Verification items for the finished model (mm, model axes). Face numbers are marked on the shaded views. A direction names the side the tool comes from. Round coordinates to 2 decimals unless told otherwise and drop trailing zeros. Order: outer loops, then holes, each group sorted by start corner. A loop starts at its lowest first (then second) coordinate and runs counter-clockwise, first axis right, second up. Notation, with made-up numbers: (47.5, 3.5) -> (67.5, 3.5) arc R18 cw to (67.5, 13.5) -> close; hole circle Ø6 at (43, 9). An arc over 180 degrees is marked (long way). Return JSON: item names as keys, results as strings. Group by question number.
Item 1: Sectioned sample at D-D on z = -12.5. Record the cut outline in (x, y) (3 decimals), plus the area to 3 significant figures.
Item 2: Depth check by flat-ended pin: pin 1 Ø1.7 at (y, z) = (12, 3) entering from +X; pin 2 Ø12 at (y, z) = (-6.5, -9.5) entering from -X (3 decimals); pin 3 Ø6 at (x, z) = (0, -13.14) entering from +Y (3 decimals); pin 4 Ø3 at (x, z) = (-10, -3) entering from -Y. Enter the tip coordinate at first touch or a pass-through.
Item 3: Sectioned sample at B-B on y = 1.5. Give the number of separate pieces and of enclosed holes in the cut face, plus the area to 3 significant figures.
Item 4: Scan lines: probe 1 along Z at (x, y) = (0, 0.5); probe 2 along X at (y, z) = (-2, -12) (3 decimals); probe 3 along Z at (x, y) = (-3, -11.5). Record each from-to range of solid material in increasing order. Write a range as from..to.
Item 5: Draft check along Z on the marked faces 1, 2, 3 and 4. Enter one of: pulls with the +Z half, pulls with the -Z half, needs draft (parallel to the pull), parting line crosses it, or undercut.
Item 6: Access from +Z, -Z, +X, -X, +Y, -Y to the whole of each face (thin tool, end or side, straight path). Record for the marked faces 5, 6 and 7.
Item 7: Sectioned sample at A-A on z = -2.75. Record the cut outline in (x, y) (3 decimals).
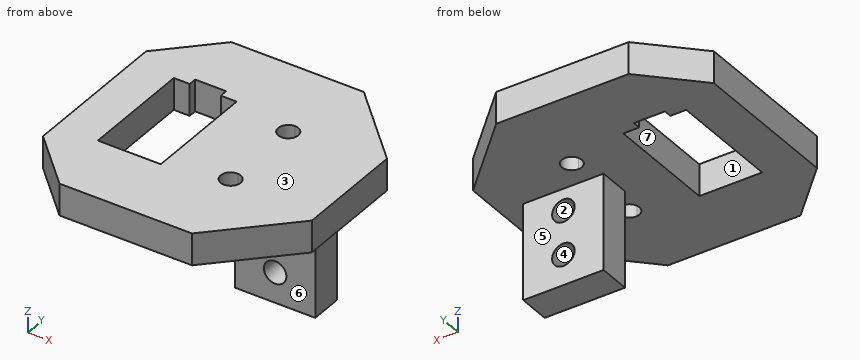
Autodesk Inventor part; units mm, degrees
ref_plane "YZ Plane" through (0, 0, 0) normal (1, 0, 0) x (0, 1, 0)
ref_plane "XZ Plane" through (0, 0, 0) normal (0, 1, 0) x (-1, 0, 0)
ref_plane "XY Plane" through (0, 0, 0) normal (0, 0, 1) x (1, 0, 0)
sketch "Sketch1" plane through (0, 0, 0) normal (0, 0, 1) x (1, 0, 0)
  line L0 (-38.1, -25.4) -> (38.1, -25.4)
  line L1 (38.1, -25.4) -> (38.1, 25.4)
  line L2 (38.1, 25.4) -> (-38.1, 25.4)
  line L3 (-38.1, 25.4) -> (-38.1, -25.4)
  line L4 (-38.1, -25.4) -> (38.1, 25.4) construction
  line L5 (38.1, -25.4) -> (-38.1, 25.4) construction
  point P0 (0, 0)
  dimension "d0" = 76.2
  dimension "d1" = 50.8
extrude "Extrusion1" add sketch "Sketch1" along normal blind 6.35
sketch "Sketch3" plane through (38.1, -25.4, 0) normal (1, 0, 0) x (0, 0, -1)
  line L0 (0, 0) -> (0, 50.8)
  line L1 (0, 50.8) -> (-6.35, 50.8)
  line L2 (-6.35, 0) -> (-6.35, 50.8)
  line L3 (0, 0) -> (-6.35, 0)
  point P0 (0, 25.4)
extrude "Extrusion3" cut sketch "Sketch3" against normal blind 25.4
sketch "Sketch4" plane through (-38.1, -25.4, 0) normal (-1, 0, 0) x (0, 0, 1)
  line L0 (4.925, 17.15) -> (1.425, 17.15)
  line L1 (1.425, 17.15) -> (1.425, 33.65)
  line L2 (1.425, 33.65) -> (4.925, 33.65)
  line L3 (4.925, 33.65) -> (4.925, 17.15)
  line L4 (4.925, 17.15) -> (1.425, 33.65) construction
  line L5 (1.425, 17.15) -> (4.925, 33.65) construction
  point P0 (0, 25.4)
  point P1 (3.175, 25.4)
  dimension "d9" = 3.5
  dimension "d10" = 16.5
extrude "Extrusion4" add sketch "Sketch4" along normal blind 3.302
sketch "Sketch5" plane through (-38.1, -8.25, 4.925) normal (0, 0, 1) x (1, 0, 0)
  line L0 (-3.302, 0) -> (-3.302, 16.5)
  line L1 (0, 16.5) -> (0, 0)
  line L2 (0, 16.5) -> (-3.302, 16.5)
  line L3 (-3.302, 0) -> (-3.302, 16.5)
  line L4 (0, 0) -> (-3.302, 0)
  line L5 (-3.302, 16.5) -> (-3.175, 16.5)
  line L6 (0, 16.5) -> (-3.302, 16.5)
  line L7 (-3.175, 16.5) -> (-3.175, 16.5685)
  line L8 (-3.302, 16.5) -> (-3.302, 0)
  line L9 (-3.175, 16.5685) -> (-3.302, 16.5)
  point P0 (38.1, 8.25)
  point P1 (-3.175, 16.5)
  dimension "d13" = 0.127
sketch3d "3D Sketch1"
  line L0 (-41.402, 8.25, 4.925) -> (-41.402, 8.25, 1.425)
  line L1 (-41.402, 8.25, 1.425) -> (-41.402, -8.25, 1.425)
  line L2 (-41.402, -8.25, 1.425) -> (-41.402, -8.25, 4.925)
  line L3 (-41.402, -8.25, 4.925) -> (-41.402, 8.25, 4.925)
sweep "Sweep1" add profiles "Sketch5" path "3D Sketch1" contours L9 L7 L2
chamfer "Chamfer1" distance 14.2875 angle 45 4 edges at (-38.1, -25.4, 3.175) (-38.1, 25.4, 3.175) (12.7, -25.4, 3.175) (12.7, 25.4, 3.175)
sketch "Sketch6" plane through (-41.402, -25.4, 0) normal (-1, 0, 0) x (0, 0, 1)
  line L0 (-26.5368, -66.9991) -> (26.5368, -66.9991)
  line L1 (26.5368, -66.9991) -> (26.5368, 66.9991)
  line L2 (26.5368, 66.9991) -> (-26.5368, 66.9991)
  line L3 (-26.5368, 66.9991) -> (-26.5368, -66.9991)
  line L4 (0, 0) -> (6.35, 0)
  line L5 (-26.5368, -66.9991) -> (26.5368, 66.9991) construction
  line L6 (26.5368, -66.9991) -> (-26.5368, 66.9991) construction
  point P0 (0, 25.4)
extrude "Extrusion5" cut sketch "Sketch6" against normal blind 28.575
sketch "Sketch7" plane through (0, 0, 0) normal (0, 0, -1) x (-1, 0, 0)
  line L0 (-8.025, 3.175) -> (-8.025, -3.175)
  line L1 (-8.025, -3.175) -> (8.025, -3.175)
  line L2 (8.025, -3.175) -> (8.025, 3.175)
  line L3 (8.025, 3.175) -> (-8.025, 3.175)
  line L4 (-8.025, 4.675) -> (8.025, -1.675) construction
  line L5 (-8.025, -1.675) -> (8.025, 4.675) construction
  line L6 (0, 3.175) -> (0, -3.175)
  point P0 (0, 0)
  point P1 (0, 0)
  dimension "d21" = 6.35
  dimension "d22" = 16.05
extrude "Extrusion6" add sketch "Sketch7" along normal blind 19.2024
sketch "Sketch9" plane through (0, 0, 6.35) normal (0, 0, 1) x (1, 0, 0)
  line L0 (6.0307, -10.9832) -> (5.9693, 11.0167)
  line L1 (-6.0307, 10.9832) -> (6.0307, 10.9832)
  line L2 (6.0307, 10.9832) -> (6.0307, -10.9832)
  line L3 (6.0307, -10.9832) -> (-6.0307, -10.9832)
  line L4 (-6.0307, -10.9832) -> (-6.0307, 10.9832)
  point P0 (0, 0)
sketch "Sketch10" plane through (-12.827, -25.4, 0) normal (-1, 0, 0) x (0, 0, 1)
  line L0 (0, 0) -> (0, 50.8)
  line L1 (6.35, 0) -> (0, 0)
  line L2 (6.35, 50.8) -> (6.35, 0)
  line L3 (0, 50.8) -> (6.35, 50.8)
  point P0 (0, 25.4)
extrude "Extrusion7" add sketch "Sketch10" along normal blind 25.4
chamfer "Chamfer2" distance 10.16 angle 45 1 edges at (-38.227, 25.4, 3.175)
chamfer "Chamfer3" distance 10.16 angle 45 1 edges at (-38.227, -25.4, 3.175)
sketch "Sketch11" plane through (0, 0, 6.35) normal (0, 0, 1) x (1, 0, 0)
  line L0 (-29.728, 10.9832) -> (-17.6666, 10.9832)
  line L1 (-17.6666, -10.9832) -> (-29.728, -10.9832)
  line L2 (-29.728, -10.9832) -> (-29.728, 10.9832)
  line L3 (-17.6666, -10.9832) -> (-17.6666, 10.9832)
  line L4 (-30.998, 12.2532) -> (-16.3966, 12.2532)
  line L5 (-16.3966, 12.2532) -> (-16.3966, -12.2532)
  line L6 (-16.3966, -12.2532) -> (-30.998, -12.2532)
  line L7 (-30.998, -12.2532) -> (-30.998, 12.2532)
  line L8 (-17.6666, 10.9832) -> (-18.9366, 10.9832)
  line L9 (-29.728, 10.9832) -> (-28.458, 10.9832)
  line L10 (-18.9366, 10.9832) -> (-28.458, 10.9832)
  line L11 (-28.458, 10.9832) -> (-28.458, 15.1856)
  line L12 (-28.458, 15.1856) -> (-18.9366, 15.1856)
  line L13 (-18.9366, 15.1856) -> (-18.9366, 10.9832)
  point P0 (0, 0)
  dimension "d54" = 1.27
  dimension "d55" = 1.27
  dimension "d56" = 1.27
extrude "Extrusion8" cut sketch "Sketch11" against normal up to surface (6.35 mm away) contours L0 L3 L1 L2
sketch "Sketch12" plane through (0, 0, 6.35) normal (0, 0, 1) x (1, 0, 0)
  arc A0 (-5.2182, -6.4143) -> (-5.5402, -10.4006) centre (-5.418, -8.4043) ccw
  arc A1 (-5.5402, -10.4006) -> (-5.2182, -6.4143) centre (-5.3404, -8.4106) ccw
  arc A2 (-5.3792, 10.6071) -> (-5.3792, 6.6078) centre (-5.418, 8.6074) ccw
  arc A3 (-5.3792, 6.6078) -> (-5.3792, 10.6071) centre (-5.3404, 8.6074) ccw
  line L0 (-14.078, 16.1258) -> (3.242, 16.1258)
  line L1 (-14.078, 16.1258) -> (-14.078, -15.929)
  line L2 (-14.078, -15.929) -> (3.242, -15.929)
  line L3 (3.242, 16.1258) -> (3.242, -15.929)
  circle A4 centre (-5.3404, -8.4106) radius 2
  circle A5 centre (-5.3404, 8.6074) radius 2
  point P0 (0, 0)
  point P1 (-5.3792, 6.6078)
  point P2 (-5.2182, -6.4143)
  point P3 (-5.5402, -10.4006)
  dimension "d38" = 4
  dimension "d39" = 4
extrude "Extrusion9" cut sketch "Sketch12" against normal up to surface (6.35 mm away) contours A1 A4 | A3 A5
sketch "Sketch13" plane through (-8.025, 3.175, 0) normal (0, 1, 0) x (1, 0, 0)
  line L0 (16.05, 19.2024) -> (0, 19.2024)
  circle A0 centre (8.025, 4.3815) radius 2.25
  circle A1 centre (8.025, 13.1445) radius 2.25
  line L1 (16.05, 0) -> (0, 0)
  line L2 (16.05, 0) -> (16.05, 19.2024)
  line L3 (0, 19.2024) -> (16.05, 19.2024)
  line L4 (0, 0) -> (0, 19.2024)
  line L5 (8.025, 0) -> (12.4065, 0)
  line L6 (6.4375, 0) -> (20.725, 0)
  line L7 (8.025, 0) -> (8.025, 4.3815)
  line L8 (8.025, 0) -> (12.4065, 0) construction
  line L9 (8.025, 0) -> (21.1695, 0)
  line L10 (8.025, 0) -> (8.025, 13.1445)
  line L11 (16.05, 0) -> (0, 0)
  line L12 (8.025, 0) -> (21.1695, 0) construction
  dimension "d44" = 4.5
  dimension "d45" = 4.5
  dimension "d48" = 4.3815
  dimension "d49" = 4.3815
  dimension "d50" = 90
  dimension "d51" = 13.1445
  dimension "d52" = 13.1445
  dimension "d53" = 90
extrude "Extrusion10" cut sketch "Sketch13" against normal up to surface (6.35 mm away) contours A1 | A0 L10 L7 | L7 L10 A0
sketch "Sketch14" plane through (0, 0, -19.2024) normal (0, 0, -1) x (-1, 0, 0)
  line L0 (8.025, 3.175) -> (8.025, -3.175)
  line L1 (-8.025, -3.175) -> (-8.025, 3.175)
  line L2 (8.025, 3.175) -> (-8.025, 3.175)
  line L3 (-8.025, 3.175) -> (-8.025, -3.175)
  line L4 (-8.025, -3.175) -> (8.025, -3.175)
  line L5 (8.025, -3.175) -> (8.025, 3.175)
  point P0 (0, 0)
sketch "Sketch16" plane through (0, 0, 6.35) normal (0, 0, 1) x (1, 0, 0)
  line L0 (-29.728, -10.9832) -> (-29.728, 10.9832)
  line L1 (-17.6666, -10.9832) -> (-29.728, -10.9832)
  line L2 (-17.6666, 10.9832) -> (-17.6666, -10.9832)
  line L3 (-29.728, 10.9832) -> (-17.6666, 10.9832)
  line L4 (-29.982, -11.2372) -> (-29.982, 11.2372)
  line L5 (-29.982, 11.2372) -> (-17.4126, 11.2372)
  line L6 (-17.4126, 11.2372) -> (-17.4126, -11.2372)
  line L7 (-17.4126, -11.2372) -> (-29.982, -11.2372)
  point P0 (0, 0)
  dimension "d62" = 0.254
extrude "Extrusion12" cut sketch "Sketch16" against normal up to surface (6.35 mm away)
sketch "Sketch17" plane through (0, 0, 6.35) normal (0, 0, 1) x (1, 0, 0)
  line L0 (-17.4126, 11.2372) -> (-29.982, 11.2372)
  line L1 (-29.982, 11.2372) -> (-26.807, 11.2372)
  line L2 (-17.4126, 11.2372) -> (-20.5876, 11.2372)
  line L3 (-26.807, 11.2372) -> (-20.5876, 11.2372)
  line L4 (-20.5876, 11.2372) -> (-20.5876, 12.8247)
  line L5 (-20.5876, 12.8247) -> (-26.807, 12.8247)
  line L6 (-26.807, 12.8247) -> (-26.807, 11.2372)
  point P0 (0, 0)
  dimension "d65" = 3.175
  dimension "d66" = 3.175
  dimension "d67" = 1.5875
extrude "Extrusion13" cut sketch "Sketch17" against normal up to surface (6.35 mm away)
properties part number "Servo Holder Module"
Recorded:
{
 "1": {"outline": "(-8.025, -3.175) -> (-2.156, -3.175) -> (-2.156, 3.175) -> (-8.025, 3.175) -> close; (2.156, -3.175) -> (8.025, -3.175) -> (8.025, 3.175) -> (2.156, 3.175) -> close", "area": "74.5 mm²"},
 "2": {"pin 1": "x = 12.66", "pin 2": "x = -8.025", "pin 3": "y = 3.175", "pin 4": "through"},
 "3": {"separate pieces": "2", "enclosed holes": "2", "area": "520 mm²"},
 "4": {"probe 1": "-19.2..-15.39, -10.89..-6.63, -2.13..6.35", "probe 2": "-8.025..-1.937, 1.937..8.025", "probe 3": "0..6.35"},
 "5": {"face 1": "needs draft", "face 2": "undercut", "face 3": "pulls with the +Z half", "face 4": "undercut"},
 "6": {"face 5": "-Z, +X, -X, +Y", "face 6": "-Z, +X, -X, -Y", "face 7": "+Z, -Z"},
 "7": {"outline": "(-8.025, -3.175) -> (-1.549, -3.175) -> (-1.549, 3.175) -> (-8.025, 3.175) -> close; (1.549, -3.175) -> (8.025, -3.175) -> (8.025, 3.175) -> (1.549, 3.175) -> close"}
}
